Read the model definition and answer for the solid it produces. Units are mm, in the model's axes. Give positions to 0.01 mm unless a question says otherwise; leave off trailing zeros. Loops run counter-clockwise (first coordinate to the right, second up) from the corner with the lowest first, then second, coordinate; pieces in that order, holes last.
(1) Find section B-B, the plane x = 14.75. Write down the section's boundary in (y, z), then the cut area to 3 significant figures.
(2) Each of these flat-tipped pins is pushed along its axis until it touches: P1, Ø2, axis at x = 19, z = 16.5, coming from the +Y side; P2, Ø6, axis at x = 23.5, z = 14, coming from the +Y side. Where does it stop, or does it pass through?
(3) Straight lines are drawn through the part: probe 1 along Y at (x, z) = (14.75, 17.25); probe 2 along Y at (x, z) = (5.25, 20.5). For each, find the intervals that lie inside material, in ascending order.
(4) Find section A-A, the plane z = 16.75. Write down the section's boundary in (x, y).
```python
from build123d import *

# Parameters (mm, degrees)
SKETCH_1_W          = 30
SKETCH_1_H          = 30
EXTRUDE_1_DEPTH     = 600
CUT_EXTRUDE_1_REACH = 603.498
CUT_EXTRUDE_2_REACH = 603.498
EXTRUDE_2_DEPTH     = 30
CUT_EXTRUDE_3_DEPTH = 30


with BuildPart() as part:
    # 草图1 → 凸台-拉伸1 (new body)
    with BuildSketch(Plane(origin=(0, 0, 0), x_dir=(1, 0, 0), z_dir=(0, 1, 0))):
        with Locations((15, -15)):
            Rectangle(SKETCH_1_W, SKETCH_1_H)
    extrude(amount=EXTRUDE_1_DEPTH)

    # 草图2 → 切除-拉伸1 (cut, up to next)
    with BuildSketch(Plane.XY.offset(30), mode=Mode.PRIVATE) as cut_extrude_1_sk1:
        Polygon((0, 0), (30, 8.038475773), (30, 0), align=None)
    cut_extrude_1_tool1 = extrude(cut_extrude_1_sk1.sketch, amount=-CUT_EXTRUDE_1_REACH, mode=Mode.PRIVATE) & part.part
    add(cut_extrude_1_tool1.solids().sort_by_distance((20, 2.679492, 30))[0], mode=Mode.SUBTRACT)

    # 草图3 → 切除-拉伸2 (cut, up to next)
    with BuildSketch(Plane(origin=(0, 0, 0), x_dir=(-1, 0, 0), z_dir=(0, 0, -1)), mode=Mode.PRIVATE) as cut_extrude_2_sk1:
        Polygon((0, 600), (-30, 600), (-30, 488.038475773), align=None)
    cut_extrude_2_tool1 = extrude(cut_extrude_2_sk1.sketch, amount=-CUT_EXTRUDE_2_REACH, mode=Mode.PRIVATE) & part.part
    add(cut_extrude_2_tool1.solids().sort_by_distance((20, 562.679492, 0))[0], mode=Mode.SUBTRACT)

    # 草图4 → 凸台-拉伸2 (add)
    with BuildSketch(Plane.XY.offset(30)):
        Polygon((0, 600), (0, -519.62), (30, -519.62), (30, 488.038475773), align=None)
    extrude(amount=-EXTRUDE_2_DEPTH)

    # 草图5 → 切除-拉伸3 (cut)
    with BuildSketch(Plane.XY.offset(30)):
        Polygon((0, 600), (0, 540), (30, 488.038475773), align=None)
    extrude(amount=-CUT_EXTRUDE_3_DEPTH, mode=Mode.SUBTRACT)


solid = part.part
```
Entries:
1. outline: (-519.62, 0) - (514.45, 0) - (514.45, 30) - (-519.62, 30) - close
1. area: 31,000 mm2
2. P1: stops at y = 508.82
2. P2: stops at y = 504.49
3. probe 1: y = -519.62 to 514.45
3. probe 2: y = -519.62 to 530.91
4. outline: (0, -519.62) - (30, -519.62) - (30, 488.04) - (0, 540) - close
